from build123d import *

# Parameters (mm, degrees)
BOSS_EXTRUDE1_DEPTH = 2.6


with BuildPart() as part:
    # Model → Boss-Extrude1 (new body)
    with BuildSketch(Plane.XY):
        with BuildLine():
            Line((-97.5, -43.8), (-93.5, -43.8))
            Line((-93.5, -43.8), (-93.5, 43.8))
            Line((-93.5, 43.8), (-97.5, 43.8))
            ThreePointArc((-97.5, 43.8), (-99.267766953, 44.532233047), (-100, 46.3))
            Line((-100, 46.3), (-100, 66.7))
            ThreePointArc((-100, 66.7), (-99.267766953, 68.467766953), (-97.5, 69.2))
            Line((-97.5, 69.2), (-93.5, 69.2))
            Line((-93.5, 69.2), (-93.5, 120))
            Line((-93.5, 120), (93.5, 120))
            Line((93.5, 120), (93.5, 69.2))
            Line((93.5, 69.2), (97.5, 69.2))
            ThreePointArc((97.5, 69.2), (99.267766953, 68.467766953), (100, 66.7))
            Line((100, 66.7), (100, 46.3))
            ThreePointArc((100, 46.3), (99.267766953, 44.532233047), (97.5, 43.8))
            Line((97.5, 43.8), (93.5, 43.8))
            Line((93.5, 43.8), (93.5, -43.8))
            Line((93.5, -43.8), (97.5, -43.8))
            ThreePointArc((97.5, -43.8), (99.267766953, -44.532233047), (100, -46.3))
            Line((100, -46.3), (100, -66.7))
            ThreePointArc((100, -66.7), (99.267766953, -68.467766953), (97.5, -69.2))
            Line((97.5, -69.2), (93.5, -69.2))
            Line((93.5, -69.2), (93.5, -120))
            Line((93.5, -120), (-93.5, -120))
            Line((-93.5, -120), (-93.5, -69.2))
            Line((-93.5, -69.2), (-97.5, -69.2))
            ThreePointArc((-97.5, -69.2), (-99.267766953, -68.467766953), (-100, -66.7))
            Line((-100, -66.7), (-100, -46.3))
            ThreePointArc((-100, -46.3), (-99.267766953, -44.532233047), (-97.5, -43.8))
        make_face()
    extrude(amount=BOSS_EXTRUDE1_DEPTH)


solid = part.part
Here's how the part is built. I have some questions about the finished solid (model axes, mm). Give positions to 0.01 mm unless a question says otherwise; leave off trailing zeros. Order: outer loops, then holes, each group sorted by start corner. A loop starts at its lowest first (then second) coordinate and runs counter-clockwise, first axis right, second up. Notation, with made-up numbers: M -19,13 L 0,13 A26 ccw 0,28 Z; hole C 69.25,21 d1. An arc over 180 degrees is marked long. Answer as a JSON object with one key per item and string values. Group by question number.
1) Suppose I cut it at A-A, the plane z = 2.05. Write out the boundary of the cut face in (x, y), plus the area to 3 significant figures.
2) Suppose I cut it at B-B, the plane y = -95. Write out the boundary of the cut face in (x, z), plus the area to 3 significant figures.
3) Please list where this line runs through material, in increasing order: L1, parallel to X at y = 40.5, z = 1.05. Write a range as [from, to].
4) I'm going to push flat-ended pins straight in: pin 1 Ø0.8 at (y, z) = (93.5, 1) entering from +X; pin 2 Ø1.3 at (x, z) = (95.5, 1.5) entering from -Y; pin 3 Ø0.8 at (x, z) = (96, 1) entering from +Y; pin 4 Ø3 at (x, y) = (-75.5, -15.5) entering from -Z. Where does each tip first touch, or does it pass through?
Results found:
{
 "1": {"outline": "M -100,-66.7 A2.5 ccw -97.5,-69.2 L -93.5,-69.2 L -93.5,-120 L 93.5,-120 L 93.5,-69.2 L 97.5,-69.2 A2.5 ccw 100,-66.7 L 100,-46.3 A2.5 ccw 97.5,-43.8 L 93.5,-43.8 L 93.5,43.8 L 97.5,43.8 A2.5 ccw 100,46.3 L 100,66.7 A2.5 ccw 97.5,69.2 L 93.5,69.2 L 93.5,120 L -93.5,120 L -93.5,69.2 L -97.5,69.2 A2.5 ccw -100,66.7 L -100,46.3 A2.5 ccw -97.5,43.8 L -93.5,43.8 L -93.5,-43.8 L -97.5,-43.8 A2.5 ccw -100,-46.3 Z", "area": "45,500 mm²"},
 "2": {"outline": "M -93.5,0 L 93.5,0 L 93.5,2.6 L -93.5,2.6 Z", "area": "486 mm²"},
 "3": {"L1": "[-93.5, 93.5]"},
 "4": {"pin 1": "x = 93.5", "pin 2": "y = -69.2", "pin 3": "y = 69.2", "pin 4": "z = 0"}
}
